```python
from build123d import *

# Parameters (mm, degrees)
EXTRUDE_THIN1_DEPTH = 10
SKETCH2_R           = 2
SKETCH2_R_2         = 2.5
CUT_EXTRUDE1_DEPTH  = 38.619808612
FILLET2_R           = 1


with BuildPart() as part:
    # Sketch1 → Extrude-Thin1 (new body)
    with BuildSketch(Plane.XY):
        Polygon((0, 0), (15, 0), (15, 8), (35, 8), (35, 6.5), (16.5, 6.5), (16.5, -1.5), (0, -1.5), align=None)
    extrude(amount=EXTRUDE_THIN1_DEPTH)

    # Sketch2 → Cut-Extrude1 (cut, through all)
    with BuildSketch(Plane(origin=(0, 8, 0), x_dir=(1, 0, 0), z_dir=(0, 1, 0))):
        with Locations(Location((30, -5, 0), (0, 0, 270))):
            Circle(SKETCH2_R)
        with Locations(Location((7.5, -5, 0), (0, 0, 270))):
            Circle(SKETCH2_R_2)
    extrude(amount=-CUT_EXTRUDE1_DEPTH, mode=Mode.SUBTRACT)

    # Fillet2
    fillet2_edges = [part.edges().sort_by_distance(p)[0] for p in [
        (16.5, 6.5, 5),
        (16.5, -1.5, 5),
        (15, 0, 5),
        (15, 8, 5),
        (0, -0.75, 10),
        (0, -0.75, 0),
        (35, 7.25, 10),
        (35, 7.25, 0),
    ]]
    fillet(fillet2_edges, radius=FILLET2_R)


solid = part.part
```
Read the model definition and answer for the solid it produces. Units are mm, in the model's axes. A direction names the side the tool comes from. Give positions to 0.01 mm unless a question says otherwise; leave off trailing zeros. Order: outer loops, then holes, each group sorted by start corner. A loop starts at its lowest first (then second) coordinate and runs counter-clockwise, first axis right, second up. Notation, with made-up numbers: (-17.5, -22.75) -> (32.5, -22.75) arc R14 ccw to (32.5, 4.25) -> close; hole circle Ø9 at (0.5, -10). An arc over 180 degrees is marked (long way). Write item = value, one per line.
1. Given pin 1 (1.8 mm diameter, centred on y = 3, z = 6, fed in from -X); pin 2 (1.8 mm diameter, centred on y = 1.5, z = 4, fed in from +X); pin 3 (3 mm diameter, centred on x = 9, y = 1, fed in from +Z); pin 4 (1.5 mm diameter, centred on x = 18, y = 1.5, fed in from -Z), each flat-ended and moving along its own axis, determine where each tip first touches the part or whether it passes through.
Numbers:
pin_1 = 15
pin_2 = 16.5
pin_3 = 10
pin_4 = through
2. A cutting plane is placed at D-D, the plane y = 3.75. Write down the section's boundary in (x, z), and give its area (3 significant figures).
Numbers:
outline = (15, 0) -> (16.5, 0) -> (16.5, 10) -> (15, 10) -> close
area = 15.0 mm²
3. A cutting plane is placed at C-C, the plane z = 8.5. Write down the section's boundary in (x, y).
Numbers:
outline = (0, -1.5) -> (15.5, -1.5) arc R1 ccw to (16.5, -0.5) -> (16.5, 5.5) arc R1 cw to (17.5, 6.5) -> (35, 6.5) -> (35, 8) -> (16, 8) arc R1 ccw to (15, 7) -> (15, 1) arc R1 cw to (14, 0) -> (0, 0) -> close
4. A cutting plane is placed at B-B, the plane z = 5. Write down the section's boundary in (x, y), and give its area (3 significant figures).
Numbers:
outline = (0, -1.5) -> (5, -1.5) -> (5, 0) -> (0, 0) -> close; (10, -1.5) -> (15.5, -1.5) arc R1 ccw to (16.5, -0.5) -> (16.5, 5.5) arc R1 cw to (17.5, 6.5) -> (28, 6.5) -> (28, 8) -> (16, 8) arc R1 ccw to (15, 7) -> (15, 1) arc R1 cw to (14, 0) -> (10, 0) -> close; (32, 6.5) -> (35, 6.5) -> (35, 8) -> (32, 8) -> close
area = 51.0 mm²
5. A cutting plane is placed at A-A, the plane x = 30. Write down the section's boundary in (y, z).
Numbers:
outline = (6.5, 0) -> (8, 0) -> (8, 3) -> (6.5, 3) -> close; (6.5, 7) -> (8, 7) -> (8, 10) -> (6.5, 10) -> close
6. The mould has two halves that part along X. Classify faces 1 (the face through (5.28, -0.74, 6.15)), 2 (the face through (25, 8, 5)), 3 (the face through (15, 4, 5)): +X half, -X half, draft (parallel to the pull), parting line (faces both ways), or undercut.
Numbers:
face_1 = undercut
face_2 = draft
face_3 = -X half
7. For faces 4 (the face through (5, 0, 3)), 5 (the face through (0, -1, 5)), 6 (the face through (16.5, 3, 5)), determine the directions among +Z, -Z, +X, -X, +Y, -Y from which every point of the face is accessible in a straight line to the end or side of a thin tool.
Numbers:
face_4 = +Z, -Z, -X, +Y
face_5 = +Z, -Z, -X, +Y, -Y
face_6 = +Z, -Z, +X, -Y
8. Straight lines are drawn through the part: line 1 along Y through (x, z) = (8, 7.5); line 2 along Y through (x, z) = (22.5, 5); line 3 along X through (y, z) = (7, 8). For each, find the intervals that lie inside material, in ascending order.
Numbers:
line_1 = -1.5 to 0
line_2 = 6.5 to 8
line_3 = 15 to 35
